Design review of the part shown in the three views and the two pictorial views. Dimensions are in mm from the part's minimum x, y and z. Coordinates: 2 decimals unless noted, no trailing zeros. Loops run counter-clockwise (first coordinate to the right, second up) from the corner with the lowest first, then second, coordinate; pieces in that order, holes last. Notation, with made-up numbers: (30.5, 10) -> (58.5, 10) arc R31 ccw to (58.5, 39) -> close; hole circle Ø8 at (77, 88). An arc over 180 degrees is marked (long way). Answer in a Markdown table with one row per item.
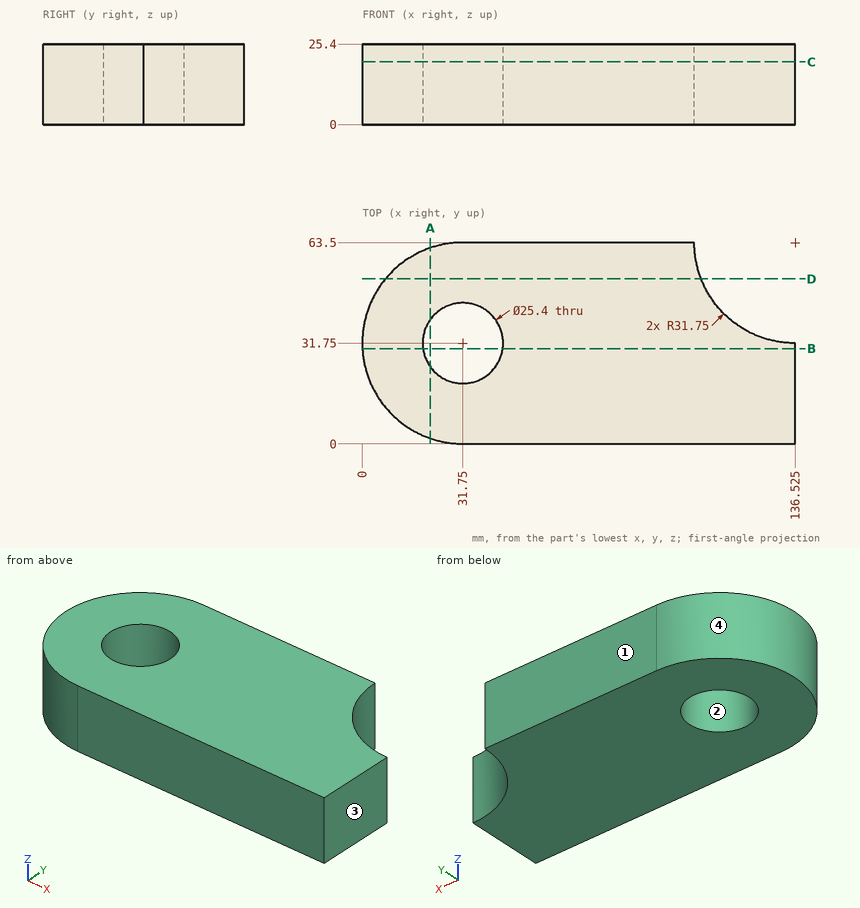
(1) Take a section at B-B on y = 30. Give the boundary of the cut face in (x, z) (3 decimals), and give its area (3 significant figures).
Evaluation:
| item | result |
|---|---|
| outline | (0.048, 0) -> (19.171, 0) -> (19.171, 25.4) -> (0.048, 25.4) -> close; (44.329, 0) -> (136.525, 0) -> (136.525, 25.4) -> (44.329, 25.4) -> close |
| area | 2,830 mm² |
(2) To check wall thickness, follow probe 1 along Y at (x, z) = (31.75, 7.75); probe 2 along X at (y, z) = (25.5, 5.5) (3 decimals); probe 3 along X at (y, z) = (28.5, 13.25) (3 decimals). State the ranges of each line that lie inside material, in increasing order.
Evaluation:
| item | result |
|---|---|
| probe 1 | y = 0 to 19.05, 44.45 to 63.5 |
| probe 2 | x = 0.621 to 20.694, 42.806 to 136.525 |
| probe 3 | x = 0.167 to 19.473, 44.027 to 136.525 |
(3) Take a section at D-D on y = 52. Give the boundary of the cut face in (x, z).
Evaluation:
| item | result |
|---|---|
| outline | (7.3, 0) -> (106.93, 0) -> (106.93, 25.4) -> (7.3, 25.4) -> close |
(4) Take a section at C-C on z = 19.75. Give the boundary of the cut face in (x, y) (3 decimals), and give its area (3 significant figures).
Evaluation:
| item | result |
|---|---|
| outline | (31.75, 0) -> (136.525, 0) -> (136.525, 31.75) arc R31.75 cw to (104.775, 63.5) -> (31.75, 63.5) arc R31.75 ccw to start; hole circle Ø25.4 at (31.75, 31.75) |
| area | 6,940 mm² |
(5) For pin 1 (6 mm diameter, centred on y = 44, z = 15.5, fed in from +X); pin 2 (5 mm diameter, centred on y = 29.5, z = 12.5, fed in from -X); pin 3 (10 mm diameter, centred on x = 20.5, z = 6, fed in from -Y), all flat-tipped, find the tip position at first contact; note any pin that passes through.
Evaluation:
| item | result |
|---|---|
| pin 1 | stops at x = 114.12 |
| pin 2 | stops at x = 0 |
| pin 3 | stops at y = 0.62 |
(6) Draft analysis for pull direction Y (two halves, no side actions). For the marked faces 1, 2, 3 and 4, state which applies: pulls with the +Y half, pulls with the -Y half, needs draft (parallel to the pull), parting line crosses it, or undercut.
Evaluation:
| item | result |
|---|---|
| face 1 | pulls with the +Y half |
| face 2 | undercut |
| face 3 | needs draft |
| face 4 | parting line crosses it |
(7) Take a section at A-A on x = 21.5. Give the boundary of the cut face in (y, z).
Evaluation:
| item | result |
|---|---|
| outline | (1.7, 0) -> (24.25, 0) -> (24.25, 25.4) -> (1.7, 25.4) -> close; (39.25, 0) -> (61.8, 0) -> (61.8, 25.4) -> (39.25, 25.4) -> close |
